Can you work these out from the model? Positions are in its coordinate system, mm. A direction names the side the tool comes from. Give positions to 0.01 mm unless a question says otherwise; leave off trailing zeros. Order: outer loops, then holes, each group sorted by start corner. A loop starts at its lowest first (then second) coordinate and runs counter-clockwise, first axis right, second up. Notation, with made-up numbers: (28.5, 23) - (53.5, 23) arc R28 ccw to (53.5, 41) - close; hole circle Ø4 at (66.25, 81). An arc over 180 degrees is marked (long way). Return JSON: item names as keys, results as strings.
```python
from build123d import *

# Parameters (mm, degrees)
SKETCH1_W                   = 50.8
SKETCH1_H                   = 25.4
SKETCH1_W_2                 = 44.45
SKETCH1_H_2                 = 19.05
BOSS_EXTRUDE1_DEPTH         = 850.9
CUT_EXTRUDE1_DEPTH          = 853.793415781
CUT_EXTRUDE1_DEPTH_BACK     = 853.793415781
SKETCH2_R                   = 3.175
F_1_4_0_25_DIAMETER_HOLE3_D = 6.35


with BuildPart() as part:
    # Sketch1 → Boss-Extrude1 (new body)
    with BuildSketch(Plane.XY):
        with Locations((25.4, 12.7)):
            Rectangle(SKETCH1_W, SKETCH1_H)
        with Locations((25.4, 12.7)):
            Rectangle(SKETCH1_W_2, SKETCH1_H_2, mode=Mode.SUBTRACT)
    extrude(amount=BOSS_EXTRUDE1_DEPTH)

    # Sketch2 → Cut-Extrude1 (cut, two sides: drawn at the far end of the back side and taken through both)
    with BuildSketch(Plane(origin=(50.8, 0, 0), x_dir=(0, 0, -1), z_dir=(1, 0, 0)).offset(-CUT_EXTRUDE1_DEPTH_BACK)):
        with Locations(Location((-800.1, 12.7, 0), (0, 0, 180))):
            Circle(SKETCH2_R)
        with Locations(Location((-787.4, 12.7, 0), (0, 0, 180))):
            Circle(SKETCH2_R)
        with Locations(Location((-774.7, 12.7, 0), (0, 0, 180))):
            Circle(SKETCH2_R)
    extrude(amount=CUT_EXTRUDE1_DEPTH + CUT_EXTRUDE1_DEPTH_BACK, mode=Mode.SUBTRACT)

    # 1/4 (0.25) Diameter Hole3 (through all)
    with Locations(Plane(origin=(0, 25.4, 0), x_dir=(1, 0, 0), z_dir=(0, 1, 0))):
        with Locations((12.7, -12.7), (25.4, -12.7), (38.1, -12.7)):
            Hole(F_1_4_0_25_DIAMETER_HOLE3_D / 2)


solid = part.part
```
1. For pin 1 Ø8.5 at (y, z) = (12.7, 800.1) entering from +X, with a flat end and sliding along its axis, tell me the tip position at first contact or that it passes through.
Checks:
{"pin 1": "x = 50.8"}
2. Suppose I cut it at A-A (z = 77). List the corners of the cut face in (x, y) for me (3 decimals), plus the area to 3 significant figures.
Checks:
{"outline": "(0, 0) - (50.8, 0) - (50.8, 25.4) - (0, 25.4) - close; hole (3.175, 3.175) - (47.625, 3.175) - (47.625, 22.225) - (3.175, 22.225) - close", "area": "444 mm^2"}
3. If I drill on L1, parallel to X at y = 22.95, z = 12.7 (3 decimals); L2, parallel to Z at x = 12.7, y = 23 (3 decimals); L3, parallel to X at y = 14.25, z = 536.5 (3 decimals), over which ranges is the centre line in solid material (lowest first)? Write a range as [from, to].
Checks:
{"L1": "[0, 9.525], [15.875, 22.225], [28.575, 34.925], [41.275, 50.8]", "L2": "[0, 9.525], [15.875, 850.9]", "L3": "[0, 3.175], [47.625, 50.8]"}
4. Thinking about a two-plate mould opening in X: for faces 1 (the face through (0, 13, 419)), 2 (the face through (25, 3.175, 419)), 3 (the face through (50.8, 13, 419)), which applies, +X half, -X half, draft (parallel to the pull), parting line (faces both ways), or undercut?
Checks:
{"face 1": "-X half", "face 2": "undercut", "face 3": "+X half"}
5. On a 3-axis mill with a long thin cutter (end or side, diameter ignored), from which of +Z, -Z, +X, -X, +Y, -Y can I reach the whole of each face in a straight line? I mean faces 4 (the face through (25, 22.225, 419)), 5 (the face through (25, 25.4, 419)). Say none if no direction works.
Checks:
{"face 4": "+Z, -Z", "face 5": "+Z, -Z, +X, -X, +Y"}
